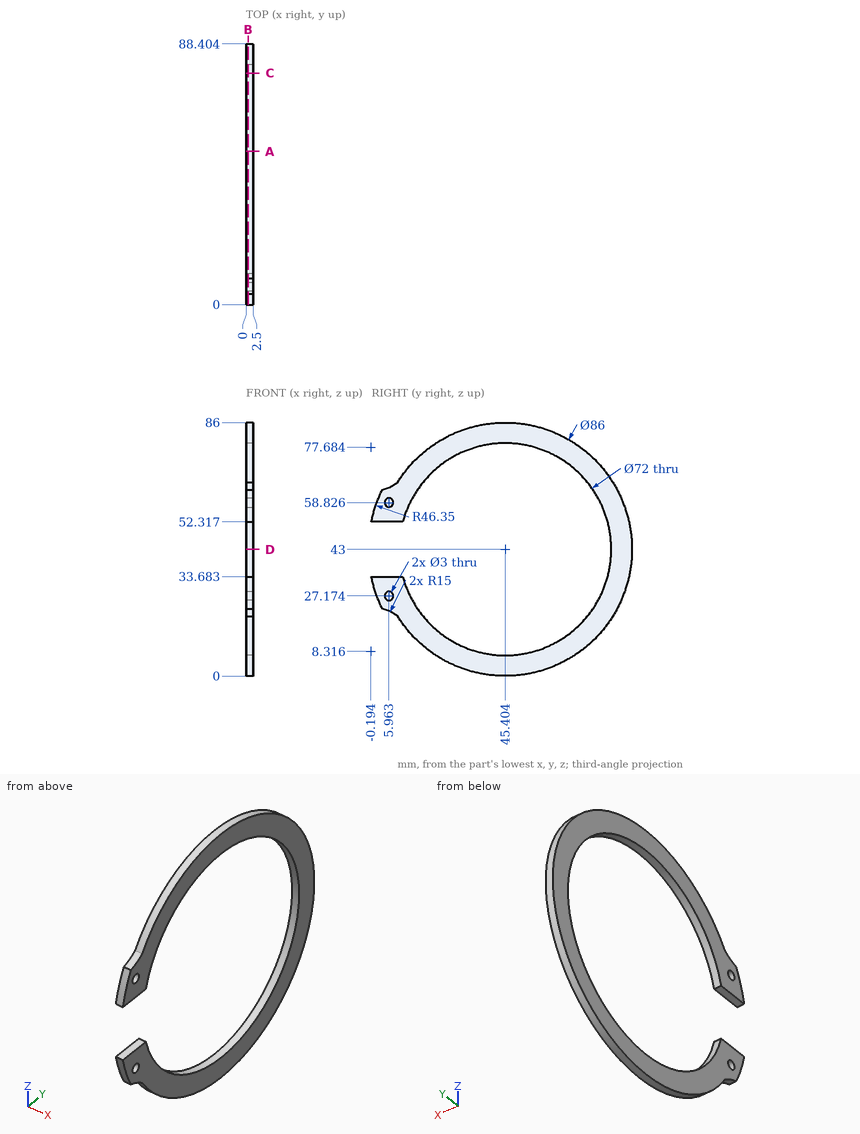
Job drawing, mm, ordinate dimensions from the low corner. One solid piece. Coordinates: 2 decimals unless noted, no trailing zeros. Write each loop counter-clockwise with the first axis right and the second up, starting at its lowest first coordinate (ties: lowest second). Pieces come first, ordered by that corner, then holes. Notation, with made-up numbers: (49, -37.5) - (95, -37.5) arc R32 cw to (95, -4.5) - close; hole circle Ø11 at (26, -21.5). An arc over 180 degrees is marked (long way). Use a Markdown table: item, result. Add a question column.
Item 1: Band-saw the part on B-B, the plane x = 0.7. Give the number of separate pieces and of enclosed holes in the cut face, and give its area (3 significant figures).
Item 2: Band-saw the part on D-D, the plane z = 43. Give the cut face in (x, y), and give its area (3 significant figures).
Item 3: Band-saw the part on A-A, the plane y = 52. Give the cut face in (x, z), and give its area (3 significant figures).
Item 4: Drill centre lines: L1, parallel to Y at x = 1.15, z = 43; L2, parallel to Z at x = 0.35, y = 59.5 (1 decimal); L3, parallel to Y at x = 0.85, z = 59.5. Where is each one in solid material? Low to high. Write a range as from..to.
Item 5: Band-saw the part on C-C, the plane y = 78.5. Give the cut face in (x, z) (1 decimal).
Item 6: Flat gauge pins, fed straight in: pin 1 (1.2 mm diameter, centred on x = 1, y = 2.5, fed in from -Z); pin 2 (12 mm diameter, centred on y = 22, z = 50.5, fed in from +X); pin 3 (0.8 mm diameter, centred on x = 1, y = 3, fed in from +Z) (1 decimal). Where does each tip first touch, or does it go through?
Numbers:
| question | item | result |
|---|---|---|
| 1 | separate pieces | 1 |
| 1 | enclosed holes | 2 |
| 1 | area | 1,680 mm2 |
| 2 | outline | (0, 81.4) - (2.5, 81.4) - (2.5, 88.4) - (0, 88.4) - close |
| 2 | area | 17.5 mm2 |
| 3 | outline | (0, 0.51) - (2.5, 0.51) - (2.5, 7.61) - (0, 7.61) - close; (0, 78.39) - (2.5, 78.39) - (2.5, 85.49) - (0, 85.49) - close |
| 3 | area | 35.5 mm2 |
| 4 | L1 | 81.4..88.4 |
| 4 | L2 | 2.4..9.9, 76.1..83.6 |
| 4 | L3 | 2.09..4.62, 7.3..13.41, 77.4..85.11 |
| 5 | outline | (0, 15.5) - (2.5, 15.5) - (2.5, 28.8) - (0, 28.8) - close; (0, 57.2) - (2.5, 57.2) - (2.5, 70.5) - (0, 70.5) - close |
| 6 | pin 1 | z = 24.06 |
| 6 | pin 2 | through |
| 6 | pin 3 | z = 62.6 |
